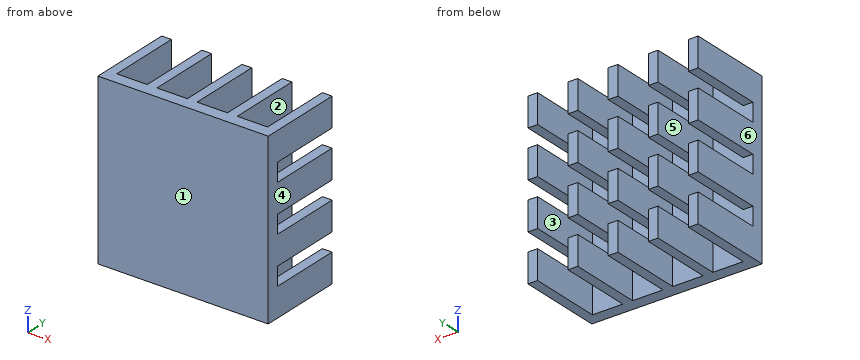
from build123d import *

# Parameters (mm, degrees)
BOSS_EXTRUDE1_DEPTH = 14
SKETCH2_W           = 1.5
SKETCH2_H           = 6
CUT_EXTRUDE1_DEPTH  = 22


with BuildPart() as part:
    # Sketch1 → Boss-Extrude1 (new body)
    with BuildSketch(Plane.XY):
        Polygon((-7, 0), (7, 0), (7, 7), (6.2, 7), (6.2, 1), (3.7, 1), (3.7, 7), (2.9, 7), (2.9, 1), (0.4, 1), (0.4, 7), (-0.4, 7), (-0.4, 1), (-2.9, 1), (-2.9, 7), (-3.7, 7), (-3.7, 1), (-6.2, 1), (-6.2, 7), (-7, 7), align=None)
    extrude(amount=BOSS_EXTRUDE1_DEPTH)

    # Sketch2 → Cut-Extrude1 (cut, through all)
    with BuildSketch(Plane.ZY.offset(7)):
        with Locations((3.125, 4)):
            Rectangle(SKETCH2_W, SKETCH2_H)
        with Locations((7, 4)):
            Rectangle(SKETCH2_W, SKETCH2_H)
        with Locations((10.875, 4)):
            Rectangle(SKETCH2_W, SKETCH2_H)
    extrude(amount=-CUT_EXTRUDE1_DEPTH, mode=Mode.SUBTRACT)


solid = part.part
Geometry check sheet. Reference: the model listing, model coordinates, mm. Face numbers are marked on the shaded views. A direction names the side the tool comes from. Give positions to 0.01 mm unless a question says otherwise; leave off trailing zeros. Loops run counter-clockwise (first coordinate to the right, second up) from the corner with the lowest first, then second, coordinate; pieces in that order, holes last. Notation, with made-up numbers: (67, -5.5) -> (94, -5.5) arc R30 ccw to (94, 30.5) -> close; hole circle Ø3 at (61, 79.25). An arc over 180 degrees is marked (long way). Answer in a Markdown table with one row per item. Add a question column.
1) Gauge pin test, flat end, axial feed: P1, Ø4, axis at x = 2, z = 5, coming from the -Y side. Record the tip position at first contact, or that the pin passes through.
2) Cross-section at B-B on z = 1.25. Record the boundary of the cut face in (x, y).
3) Cross-section at A-A on y = 6. State how many separate pieces and enclosed holes the cut face has, and give its area (3 significant figures).
4) Draft check along X on the marked faces 1, 2, 3 and 4. Enter one of: pulls with the +X half, pulls with the -X half, needs draft (parallel to the pull), parting line crosses it, or undercut.
5) Material ranges on probe 1 along X at (y, z) = (4.5, 5); probe 2 along Z at (x, y) = (6.75, 1.5) (3 decimals); probe 3 along Y at (x, z) = (5.25, 1), recorded low to high. Write a range as from..to.
6) Cross-section at C-C on x = -1.5. Record the boundary of the cut face in (y, z), and give its area (3 significant figures).
7) Set-up check for the marked faces 5 and 6: record each of +Z, -Z, +X, -X, +Y, -Y from which the full face is reachable in a straight line by a thin tool's end or side.
Outcome:
| question | item | result |
|---|---|---|
| 1 | P1 | stops at y = 0 |
| 2 | outline | (-7, 0) -> (7, 0) -> (7, 7) -> (6.2, 7) -> (6.2, 1) -> (3.7, 1) -> (3.7, 7) -> (2.9, 7) -> (2.9, 1) -> (0.4, 1) -> (0.4, 7) -> (-0.4, 7) -> (-0.4, 1) -> (-2.9, 1) -> (-2.9, 7) -> (-3.7, 7) -> (-3.7, 1) -> (-6.2, 1) -> (-6.2, 7) -> (-7, 7) -> close |
| 3 | separate pieces | 20 |
| 3 | enclosed holes | 0 |
| 3 | area | 38.0 mm^2 |
| 4 | face 1 | needs draft |
| 4 | face 2 | undercut |
| 4 | face 3 | undercut |
| 4 | face 4 | pulls with the +X half |
| 5 | probe 1 | x = -7..-6.2, -3.7..-2.9, -0.4..0.4, 2.9..3.7, 6.2..7 |
| 5 | probe 2 | z = 0..2.375, 3.875..6.25, 7.75..10.125, 11.625..14 |
| 5 | probe 3 | y = 0..1 |
| 6 | outline | (0, 0) -> (1, 0) -> (1, 14) -> (0, 14) -> close |
| 6 | area | 14.0 mm^2 |
| 7 | face 5 | +Z, -Z, +Y |
| 7 | face 6 | +Z, -Z, -X, +Y, -Y |
